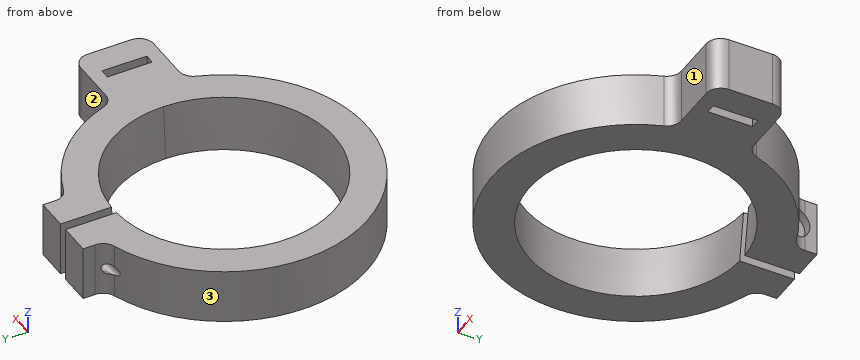
```python
from build123d import *

# Parameters (mm, degrees)
F0_R           = 49.784
F0_R_2         = 37.084
F1_DEPTH       = 19.05
F2_R           = 37.084
F3_DEPTH       = 19.05
F3_TAPER       = -4
F4_W           = 25.4
F4_H           = 17.7178942325
F5_DEPTH       = 19.05
F6_W           = 3.175
F6_H           = 19.0839946053
F7_DEPTH       = 19.0510001
F8_W           = 34.3662
F8_H           = 25.4
F9_DEPTH       = 19.05
F10_W          = 3.429
F10_H          = 15.621
F11_DEPTH      = 19.0510001
F12_R          = 2.5527
F13_DEPTH      = 11.1125
F13_DEPTH_BACK = 60.0833057675
F14_R          = 5.5245
F15_DEPTH      = 3.175
F15_DEPTH_BACK = 60.0833057675
F17_D          = 3.7973
F18_T1_DEPTH   = 19.05
F18_T6_DEPTH   = 13.4160756928
F18_S7_R       = 5.5245
F18_T8_DEPTH   = 9
F18_T12_DEPTH  = 13.4160756928
F18_S13_R      = 5.5245
F18_T14_DEPTH  = 9
F18_T18_DEPTH  = 17.0419256928
F18_S19_R      = 1.89865
F18_T20_DEPTH  = 11
F18_T24_DEPTH  = 17.0419256928
F18_S25_R      = 1.89865
F18_T26_DEPTH  = 11
F18_T27_DEPTH  = 44.45


# Not quite as in the source:
# - a fillet or chamfer that OpenCascade refuses, or shapes differently, is made with other operations: its cross-section is extruded or revolved along the edge and cut away or added


with BuildPart() as f1:
    # F0 (on Top) → F1 (new body)
    with BuildSketch(Plane.XY):
        Circle(F0_R)
        Circle(F0_R_2, mode=Mode.SUBTRACT)
    extrude(amount=F1_DEPTH)

    # F2 (on face) → F3 (cut)
    with BuildSketch(Plane(origin=(0, 0, 0), x_dir=(1, 0, 0), z_dir=(0, 0, -1))):
        Circle(F2_R)
    extrude(amount=-F3_DEPTH, taper=F3_TAPER, mode=Mode.SUBTRACT)

    # F4 (on face) → F5 (join)
    with BuildSketch(Plane.XY.offset(19.05)):
        with Locations((0, 47.2750528838)):
            Rectangle(F4_W, F4_H)
    extrude(amount=-F5_DEPTH)

    # F6 (on face) → F7 (cut, through all)
    with BuildSketch(Plane.XY.offset(19.05)):
        with Locations((0, 46.5920026974)):
            Rectangle(F6_W, F6_H)
    extrude(amount=-F7_DEPTH, mode=Mode.SUBTRACT)

    # F8 (on face) → F9 (join)
    with BuildSketch(Plane.XY.offset(19.05)):
        with Locations((55.5992057675, 0)):
            Rectangle(F8_W, F8_H)
    extrude(amount=-F9_DEPTH)

    # F10 (on face) → F11 (cut, through all)
    with BuildSketch(Plane.XY.offset(19.05)):
        with Locations((61.5315, 0)):
            Rectangle(F10_W, F10_H)
    extrude(amount=-F11_DEPTH, mode=Mode.SUBTRACT)

    # F12 (on face) → F13 (cut, two sides)
    with BuildSketch(Plane.YZ.offset(12.7)) as f13_sk:
        with Locations((48.1368534078, 9.525)):
            Circle(F12_R)
    extrude(amount=-F13_DEPTH, mode=Mode.SUBTRACT)
    extrude(f13_sk.sketch, amount=F13_DEPTH_BACK, mode=Mode.SUBTRACT)

    # F14 (on face) → F15 (cut, two sides)
    with BuildSketch(Plane.YZ.offset(12.7)) as f15_sk:
        with Locations((48.1368534078, 9.525)):
            Circle(F14_R)
    extrude(amount=-F15_DEPTH, mode=Mode.SUBTRACT)
    extrude(f15_sk.sketch, amount=F15_DEPTH_BACK, mode=Mode.SUBTRACT)

    # F17 (through all)
    with Locations(Plane.YZ.offset(-1.5875)):
        with Locations((48.1368534078, 9.525)):
            Hole(F17_D / 2)

    # F18: fillet of radius 5.08 on 8 edges, made by hand

    # F18_s2 → F18_t1 (join)
    with BuildSketch(Plane.XY):
        with BuildLine():
            ThreePointArc((47.0972426029, -16.1337037037), (48.949846917, -13.6466245522), (51.9030836849, -12.7))
            Line((51.9030836849, -12.7), (48.1368534078, -12.7))
            ThreePointArc((48.1368534078, -12.7), (47.6479888455, -14.4262197049), (47.0972426029, -16.1337037037))
        make_face()
        with BuildLine():
            ThreePointArc((51.9030836849, 12.7), (48.949846917, 13.6466245522), (47.0972426029, 16.1337037037))
            ThreePointArc((47.0972426029, 16.1337037037), (47.6479888455, 14.4262197049), (48.1368534078, 12.7))
            Line((48.1368534078, 12.7), (51.9030836849, 12.7))
        make_face()
    extrude(amount=F18_T1_DEPTH)


with BuildPart() as f18_tool4:
    # F18_s5 → F18_t6 (new body)
    with BuildSketch(Plane.XY.offset(13.4160756928)):
        with BuildLine():
            ThreePointArc((12.7, 51.9030836849), (13.6466245522, 48.949846917), (16.1337037037, 47.0972426029))
            ThreePointArc((16.1337037037, 47.0972426029), (14.4262197049, 47.6479888455), (12.7, 48.1368534078))
            Line((12.7, 48.1368534078), (12.7, 51.9030836849))
        make_face()
    extrude(amount=-F18_T6_DEPTH)

    # F18_s7 → F18_t8 (cut, symmetric)
    with BuildSketch(Plane.YZ.offset(14.4)):
        with Locations((48.1368534078, 9.525)):
            Circle(F18_S7_R)
    extrude(amount=F18_T8_DEPTH, both=True, mode=Mode.SUBTRACT)


with BuildPart() as f1_1:
    add(f1.part)

    # F18_t3: union F18_tool4
    add(f18_tool4.part)


with BuildPart() as f18_tool10:
    # F18_s11 → F18_t12 (new body)
    with BuildSketch(Plane.XY.offset(19.05)):
        with BuildLine():
            ThreePointArc((12.7, 51.9030836849), (13.6466245522, 48.949846917), (16.1337037037, 47.0972426029))
            ThreePointArc((16.1337037037, 47.0972426029), (14.4262197049, 47.6479888455), (12.7, 48.1368534078))
            Line((12.7, 48.1368534078), (12.7, 51.9030836849))
        make_face()
    extrude(amount=-F18_T12_DEPTH)

    # F18_s13 → F18_t14 (cut, symmetric)
    with BuildSketch(Plane.YZ.offset(14.4)):
        with Locations((48.1368534078, 9.525)):
            Circle(F18_S13_R)
    extrude(amount=F18_T14_DEPTH, both=True, mode=Mode.SUBTRACT)


with BuildPart() as f1_2:
    add(f1_1.part)

    # F18_t9: union F18_tool10
    add(f18_tool10.part)


with BuildPart() as f18_tool16:
    # F18_s17 → F18_t18 (new body)
    with BuildSketch(Plane.XY.offset(19.05)):
        with BuildLine():
            ThreePointArc((-16.1337037037, 47.0972426029), (-13.6466245522, 48.949846917), (-12.7, 51.9030836849))
            Line((-12.7, 51.9030836849), (-12.7, 48.1368534078))
            ThreePointArc((-12.7, 48.1368534078), (-14.4262197049, 47.6479888455), (-16.1337037037, 47.0972426029))
        make_face()
    extrude(amount=-F18_T18_DEPTH)

    # F18_s19 → F18_t20 (cut, symmetric)
    with BuildSketch(Plane.YZ.offset(-14.4)):
        with Locations((48.1368534078, 9.525)):
            Circle(F18_S19_R)
    extrude(amount=F18_T20_DEPTH, both=True, mode=Mode.SUBTRACT)


with BuildPart() as f1_3:
    add(f1_2.part)

    # F18_t15: union F18_tool16
    add(f18_tool16.part)


with BuildPart() as f18_tool22:
    # F18_s23 → F18_t24 (new body)
    with BuildSketch(Plane.XY.offset(17.0419256928)):
        with BuildLine():
            ThreePointArc((-16.1337037037, 47.0972426029), (-13.6466245522, 48.949846917), (-12.7, 51.9030836849))
            Line((-12.7, 51.9030836849), (-12.7, 48.1368534078))
            ThreePointArc((-12.7, 48.1368534078), (-14.4262197049, 47.6479888455), (-16.1337037037, 47.0972426029))
        make_face()
    extrude(amount=-F18_T24_DEPTH)

    # F18_s25 → F18_t26 (cut, symmetric)
    with BuildSketch(Plane.YZ.offset(-14.4)):
        with Locations((48.1368534078, 9.525)):
            Circle(F18_S25_R)
    extrude(amount=F18_T26_DEPTH, both=True, mode=Mode.SUBTRACT)


with BuildPart() as f1_4:
    add(f1_3.part)

    # F18_t21: union F18_tool22
    add(f18_tool22.part)

    # F18_s28 → F18_t27 (cut)
    with BuildSketch(Plane.XY.offset(-12.7)):
        with BuildLine():
            ThreePointArc((67.7023057675, -12.7), (71.294408216, -11.2121024484), (72.7823057675, -7.62))
            Line((72.7823057675, -7.62), (72.7823057675, -12.7))
            Line((72.7823057675, -12.7), (67.7023057675, -12.7))
        make_face()
        with BuildLine():
            ThreePointArc((72.7823057675, 7.62), (71.294408216, 11.2121024484), (67.7023057675, 12.7))
            Line((67.7023057675, 12.7), (72.7823057675, 12.7))
            Line((72.7823057675, 12.7), (72.7823057675, 7.62))
        make_face()
    extrude(amount=F18_T27_DEPTH, mode=Mode.SUBTRACT)


solid = f1_4.part
```
Can you work these out from the model? Positions are in its coordinate system, mm. Face numbers are marked on the shaded views. A direction names the side the tool comes from. Give positions to 0.01 mm unless a question says otherwise; leave off trailing zeros. Order: outer loops, then holes, each group sorted by start corner. A loop starts at its lowest first (then second) coordinate and runs counter-clockwise, first axis right, second up. Notation, with made-up numbers: M 55.25,61 L 104.25,61 A22 ccw 104.25,86 Z; hole C 7.5,41 d10. An arc over 180 degrees is marked long. One line per item, written item: value.
1) I want a section at A-A, the plane z = 16.5. List the corners of the cut face in (x, y) for me.
Answer sheet:
outline: M -16.13,47.1 A49.78 ccw long 47.1,-16.13 A5.08 cw 51.9,-12.7 L 67.7,-12.7 A5.08 ccw 72.78,-7.62 L 72.78,7.62 A5.08 ccw 67.7,12.7 L 51.9,12.7 A5.08 cw 47.1,16.13 A49.78 ccw 16.13,47.1 A5.08 cw 12.7,51.9 L 12.7,56.13 L 1.59,56.13 L 1.59,38.2 A38.24 cw long -1.59,38.2 L -1.59,56.13 L -12.7,56.13 L -12.7,51.9 A5.08 cw Z; hole M 59.82,-7.81 L 63.25,-7.81 L 63.25,7.81 L 59.82,7.81 Z
2) Please list where these lines run through material, in increasing order: line 1 along Y through (x, z) = (12, 7.5); line 2 along X through (y, z) = (0, 17.25); line 3 along Y through (x, z) = (-15.5, 3).
Answer sheet:
line 1: y = -48.32 to -35.64, 35.64 to 43, 53.28 to 56.13
line 2: x = -49.78 to -38.29, 38.29 to 59.82, 63.25 to 72.78
line 3: y = -47.31 to -33.92, 33.92 to 47.36
3) I want a section at B-B, the plane x = -9. Count the separate pieces of the cut face and the enclosed holes in it, plus the area to 3 significant figures.
Answer sheet:
separate pieces: 2
enclosed holes: 1
area: 594 mm^2
4) For P1, Ø8, axis at y = 3, z = 6, coming from the -X side; P2, Ø2.5, axis at x = 61, z = 8, coming from the +Y side; P3, Ø8, axis at x = 17, y = 26, coming from the +Z side; P4, Ø1.7, axis at x = 61, z = 5.5, coming from the -Y side, each with a flat end and sliding along its axis, tell me the tip position at first contact or that it passes through.
Answer sheet:
P1: stops at x = -49.78
P2: stops at y = 12.7
P3: passes through
P4: stops at y = -12.7
5) I want a section at D-D, the plane y = -43. List the corners of the cut face in (x, z) for me, plus the area to 3 significant figures.
Answer sheet:
outline: M -25.09,0 L 25.09,0 L 25.09,19.05 L -25.09,19.05 Z
area: 956 mm^2
6) On a 3-axis mill with a long thin cutter (end or side, diameter ignored), from which of +Z, -Z, +X, -X, +Y, -Y can I reach the whole of each face in a straight line? I mean the marked faces 1, 2 and 3. Say none if no direction works.
Answer sheet:
face 1: +Z, -Z, +X, -Y
face 2: +Z, -Z, +X, +Y
face 3: +Z, -Z
7) I want a section at C-C, the plane x = 65. List the corners of the cut face in (y, z) for me.
Answer sheet:
outline: M -12.7,0 L 12.7,0 L 12.7,19.05 L -12.7,19.05 Z
